```python
from build123d import *

# Parameters (mm, degrees)
F0_W      = 18
F0_H      = 1.25
F1_DEPTH  = 17
F2_W      = 12
F2_H      = 17
F3_DEPTH  = 1.5
F5_DEPTH  = 3
F6_W      = 4
F6_H      = 1.5
F7_DEPTH  = 0.5
F9_DEPTH  = 25
F11_DEPTH = 0.4


with BuildPart() as f1:
    # F0 (on Front) → F1 (new body)
    with BuildSketch(Plane.XZ):
        Rectangle(F0_W, F0_H)
    extrude(amount=F1_DEPTH)

    # F2 (on face) → F3 (join)
    with BuildSketch(Plane.XY.offset(0.625)):
        with Locations((0, -8.5)):
            Rectangle(F2_W, F2_H)
    extrude(amount=F3_DEPTH)

    # F4 (on face) → F5 (join)
    with BuildSketch(Plane(origin=(0, 0, 0), x_dir=(-1, 0, 0), z_dir=(0, 1, 0))):
        Polygon((-2, 0.375), (-2, -0.625), (0, -0.625), (2, -0.625), (2, 0.375), align=None)
    extrude(amount=F5_DEPTH)

    # F6 (on face) → F7 (cut)
    with BuildSketch(Plane.XY.offset(0.375)):
        with Locations((0, 0.75)):
            Rectangle(F6_W, F6_H)
    extrude(amount=-F7_DEPTH, mode=Mode.SUBTRACT)

    # F8 (on face) → F9 (cut)
    with BuildSketch(Plane(origin=(-2, 0, 0), x_dir=(0, -1, 0), z_dir=(-1, 0, 0))):
        Polygon((-3, 0.375), (-3, -0.125), (-2.5, 0.375), align=None)
    extrude(amount=-F9_DEPTH, mode=Mode.SUBTRACT)

    # F10 (on face) → F11 (cut)
    with BuildSketch(Plane.XY.offset(2.125)):
        with BuildLine():
            Line((0, -2.7756802738), (0, -1.7756802738))
            Line((0, -1.7756802738), (-2.2519526784, -1.7756802738))
            ThreePointArc((-2.2519526784, -1.7756802738), (-2.4273486216, -1.8483316522), (-2.5, -2.0237275953))
            Line((-2.5, -2.0237275953), (-2.5, -2.5276329522))
            ThreePointArc((-2.5, -2.5276329522), (-2.4273486216, -2.7030288953), (-2.2519526784, -2.7756802738))
            Line((-2.2519526784, -2.7756802738), (0, -2.7756802738))
        make_face()
        with BuildLine():
            Line((2.25, -1.7756802738), (0, -1.7756802738))
            Line((0, -1.7756802738), (0, -2.7756802738))
            Line((0, -2.7756802738), (2.2519526784, -2.7756802738))
            ThreePointArc((2.2519526784, -2.7756802738), (2.4273486216, -2.7030288953), (2.5, -2.5276329522))
            Line((2.5, -2.5276329522), (2.5, -2.0256802738))
            ThreePointArc((2.5, -2.0256802738), (2.4267766953, -1.8489035785), (2.25, -1.7756802738))
        make_face()
        Polygon((0, -14.6959666163), (0, -13.8118481482), (-2.3675321166, -7.7671974242), (-3.0425887489, -7.7671974242), (-5.7699987665, -14.6959666163), (-4.9575144977, -14.6959666163), (-4.1087855775, -12.501655013), (-1.3436207146, -12.501655013), (-0.4843204378, -14.6959666163), align=None)
        with BuildLine():
            Line((-2.396225799, -9.6413479402), (-1.592802693, -11.7797823726))
            Line((-1.592802693, -11.7797823726), (-3.8248691415, -11.7797823726))
            Line((-3.8248691415, -11.7797823726), (-3.0138950665, -9.6413479402))
            add(Edge.make_bspline(
                [(-2.7163868863, -8.6461302206), (-2.8205902591, -9.0991883631), (-3.0138950665, -9.6413479402)],
                knots=[0, 0, 0, 1, 1, 1], degree=2))
            add(Edge.make_bspline(
                [(-2.396225799, -9.6413479402), (-2.5517757612, -9.2351058058), (-2.7163868863, -8.6461302206)],
                knots=[0, 0, 0, 1, 1, 1], degree=2))
        make_face(mode=Mode.SUBTRACT)
        Polygon((2.6161074505, -14.6959666163), (3.4180203626, -14.6959666163), (3.4180203626, -8.5087025841), (5.6032708031, -8.5087025841), (5.6032708031, -7.7958911066), (0.43085701, -7.7958911066), (0.43085701, -8.5087025841), (2.6161074505, -8.5087025841), align=None)
        Polygon((0.3462861567, -14.6959666163), (0, -13.8118481482), (0, -14.6959666163), align=None)
    extrude(amount=-F11_DEPTH, mode=Mode.SUBTRACT)


solid = f1.part
```
Input: part model. Units: mm. Frame: model coordinates. A direction names the side the tool comes from. Give positions to 0.01 mm unless a question says otherwise; leave off trailing zeros. Loops run counter-clockwise (first coordinate to the right, second up) from the corner with the lowest first, then second, coordinate; pieces in that order, holes last. Notation, with made-up numbers: (21.25, 88) -> (32.25, 88) arc R33 ccw to (32.25, 116) -> close; hole circle Ø3 at (-5.5, -2.75). An arc over 180 degrees is marked (long way). Use a Markdown table: item, result.
Q1. Section query B-B, the plane z = -0.4. Return the cut outline in (x, y), plus the area to 3 significant figures.
Entries:
| item | result |
|---|---|
| outline | (-9, -17) -> (9, -17) -> (9, 0) -> (2, 0) -> (2, 3) -> (-2, 3) -> (-2, 0) -> (-9, 0) -> close |
| area | 318 mm² |
Q2. Section query A-A, the plane x = 3. Return the cut outline in (y, z) (3 decimals).
Entries:
| item | result |
|---|---|
| outline | (-17, -0.625) -> (0, -0.625) -> (0, 2.125) -> (-7.796, 2.125) -> (-7.796, 1.725) -> (-14.696, 1.725) -> (-14.696, 2.125) -> (-17, 2.125) -> close |
Q3. Section query C-C, the plane z = 0.95. Return the cut outline in (x, y).
Entries:
| item | result |
|---|---|
| outline | (-6, -17) -> (6, -17) -> (6, 0) -> (-6, 0) -> close |
Q4. Pull-direction query (Y, two-part tool) for faces 1 (the flat face through (-3, -11, 2.125)), 2 (the flat face through (-3.425, -10.726, 1.928)), 3 (the flat face through (0, -17, 1)); classes: pulls with the +Y half, pulls with the -Y half, needs draft (parallel to the pull), parting line crosses it, or undercut.
Entries:
| item | result |
|---|---|
| face 1 | needs draft |
| face 2 | undercut |
| face 3 | pulls with the -Y half |
Q5. Access query for faces 4 (the flat face through (7, -8, 0.625)), 5 (the flat face through (0, 1, -0.125)), 6 (the flat face through (-6, -9, 1)), 7 (the flat face through (-0.92, -13.58, 1.93)). Directions: +Z, -Z, +X, -X, +Y, -Y. A direction counts if a zero-diameter tool reaches every point of the face in a straight line with its end or side. Return the directions, or none.
Entries:
| item | result |
|---|---|
| face 4 | +Z, +X, +Y, -Y |
| face 5 | +Z, +X, -X |
| face 6 | +Z, -X, +Y, -Y |
| face 7 | +Z |
Q6. Ray query, probe 1 along Z at (x, y) = (-8, -1) (3 decimals); probe 2 along Y at (x, z) = (-3, 0.1); probe 3 along X at (y, z) = (-9.5, 1.2). Return the intervals inside material, ascending. Write a range as from..to.
Entries:
| item | result |
|---|---|
| probe 1 | z = -0.625..0.625 |
| probe 2 | y = -17..0 |
| probe 3 | x = -6..6 |
Q7. First-contact query: P1, Ø0.9, axis at x = 7, y = -12, coming from the +Z side (3 decimals); P2, Ø0.8, axis at x = 0, y = 2, coming from the +Z side (3 decimals). Flat tips, straight axial feed; report the tip coordinate or a pass-through.
Entries:
| item | result |
|---|---|
| P1 | stops at z = 0.625 |
| P2 | stops at z = 0.375 |
Q8. Section query D-D, the plane x = 6.5. Return the cut outline in (y, z) (3 decimals).
Entries:
| item | result |
|---|---|
| outline | (-17, -0.625) -> (0, -0.625) -> (0, 0.625) -> (-17, 0.625) -> close |
